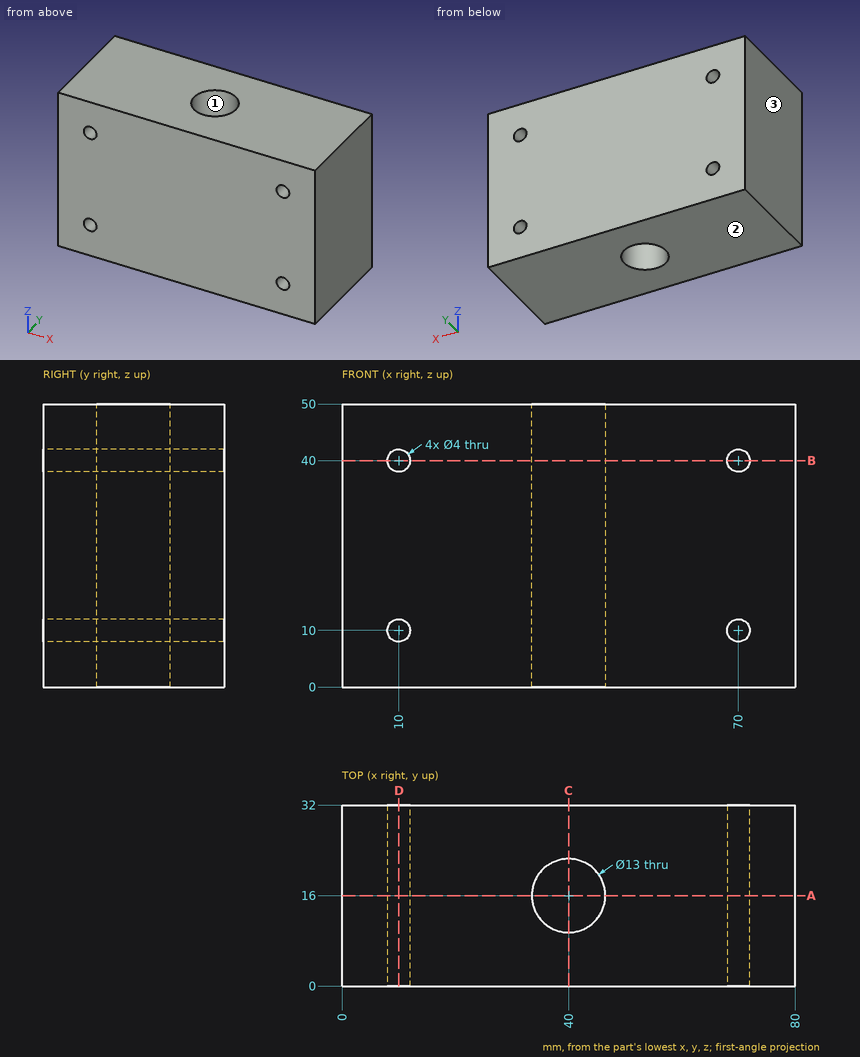
Design review of the part shown in the three views and the two pictorial views. Dimensions are in mm from the part's minimum x, y and z. Round coordinates to 2 decimals unless told otherwise and drop trailing zeros. Loops run counter-clockwise (first coordinate to the right, second up) from the corner with the lowest first, then second, coordinate; pieces in that order, holes last. Notation, with made-up numbers: (24, 26) - (62, 26) arc R29 cw to (62, 46) - close; hole circle Ø2 at (33.5, 21). An arc over 180 degrees is marked (long way). Use CSV: the item, a comma, the result in double quotes.
(1) The part is to be moulded in two halves that separate along X. For the marked faces 1, 2 and 3, say which applies: pulls with the +X half, pulls with the -X half, needs draft (parallel to the pull), parting line crosses it, or undercut.
Working result:
face 1,"undercut"
face 2,"needs draft"
face 3,"pulls with the -X half"
(2) For line 1 (Z direction, x = 70, y = 20); line 2 (X direction, y = 26.5, z = 10); line 3 (X direction, y = 23, z = 41), list the stretches that pass through material, from the lowest coordinate up.
Working result:
line 1,"z = 0 to 8, 12 to 38, 42 to 50"
line 2,"x = 0 to 8, 12 to 68, 72 to 80"
line 3,"x = 0 to 8.27, 11.73 to 68.27, 71.73 to 80"
(3) Take a section at D-D, the plane x = 10. Give the boundary of the cut face in (y, z).
Working result:
outline,"(0, 0) - (32, 0) - (32, 8) - (0, 8) - close; (0, 12) - (32, 12) - (32, 38) - (0, 38) - close; (0, 42) - (32, 42) - (32, 50) - (0, 50) - close"
(4) Take a section at B-B, the plane z = 40. Give the boundary of the cut face in (x, y), plus the area to 3 significant figures.
Working result:
outline,"(0, 0) - (8, 0) - (8, 32) - (0, 32) - close; (12, 0) - (68, 0) - (68, 32) - (12, 32) - close; (72, 0) - (80, 0) - (80, 32) - (72, 32) - close; hole circle Ø13 at (40, 16)"
area,"2,170 mm^2"
(5) Take a section at C-C, the plane x = 40. Give the boundary of the cut face in (y, z), plus the area to 3 significant figures.
Working result:
outline,"(0, 0) - (9.5, 0) - (9.5, 50) - (0, 50) - close; (22.5, 0) - (32, 0) - (32, 50) - (22.5, 50) - close"
area,"950 mm^2"
(6) Take a section at A-A, the plane y = 16. Give the boundary of the cut face in (x, z).
Working result:
outline,"(0, 0) - (33.5, 0) - (33.5, 50) - (0, 50) - close; (46.5, 0) - (80, 0) - (80, 50) - (46.5, 50) - close; hole circle Ø4 at (10, 10); hole circle Ø4 at (10, 40); hole circle Ø4 at (70, 10); hole circle Ø4 at (70, 40)"
